The figure shows three views and two pictorial views of one solid part (mm, origin at its lowest corner). Answer the questions. A direction names the side the tool comes from. Round coordinates to 2 decimals unless told otherwise and drop trailing zeros. Write each loop counter-clockwise with the first axis right and the second up, starting at its lowest first coordinate (ties: lowest second). Pieces come first, ordered by that corner, then holes.
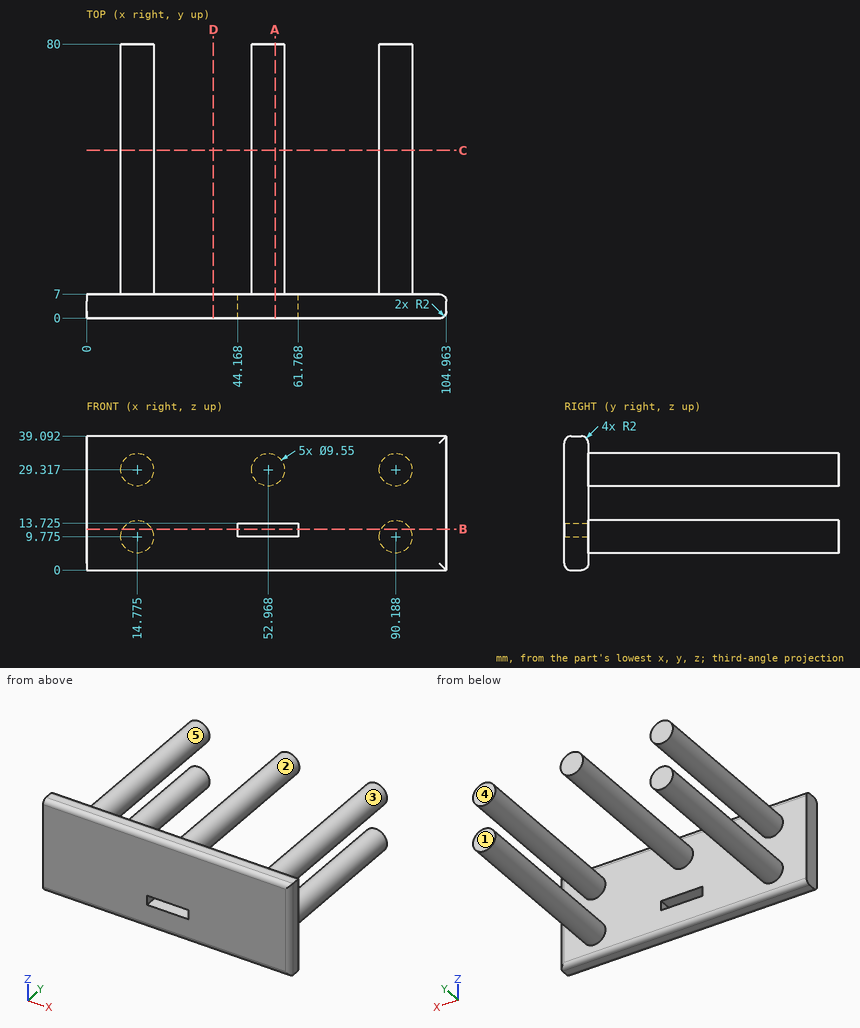
Q1. Determine the mould class of the marked faces 1, 2 and 3 for opening direction Z: pulls with the +Z half, pulls with the -Z half, needs draft (parallel to the pull), parting line crosses it, or undercut.
Verdict:
face 1: needs draft
face 2: parting line crosses it
face 3: undercut
Q2. Flat-ended cylindrical pins translate along their axes: pin 1 Ø12 at (y, z) = (28, 6) entering from +X; pin 2 Ø1 at (x, z) = (56.5, 22.5) entering from +Y; pin 3 Ø10 at (y, z) = (24, 6) entering from -X; pin 4 Ø4 at (y, z) = (38, 18.5) entering from +X. Find the tip coordinate at first contact, or state that the pin passes through.
Verdict:
pin 1: stops at x = 94.96
pin 2: stops at y = 7
pin 3: stops at x = 10
pin 4: passes through
Q3. Section B-B (z = 12) is taken. Determine the outline of the cut face in (x, y), then the cut area to 3 significant figures.
Verdict:
outline: (0, 0) - (44.17, 0) - (44.17, 7) - (19, 7) - (19, 80) - (10.55, 80) - (10.55, 7) - (0, 7) - close; (61.77, 0) - (102.96, 0) arc R2 ccw to (104.96, 2) - (104.96, 5) arc R2 ccw to (102.96, 7) - (94.41, 7) - (94.41, 80) - (85.96, 80) - (85.96, 7) - (61.77, 7) - close
area: 1,840 mm2
Q4. Section A-A (x = 55) is taken. Determine the outline of the cut face in (y, z) (1 decimal).
Verdict:
outline: (0, 2) arc R2 ccw to (2, 0) - (5, 0) arc R2 ccw to (7, 2) - (7, 9.8) - (0, 9.8) - close; (0, 13.7) - (7, 13.7) - (7, 25) - (80, 25) - (80, 33.6) - (7, 33.6) - (7, 37.1) arc R2 ccw to (5, 39.1) - (2, 39.1) arc R2 ccw to (0, 37.1) - close
Q5. Straight lines are drawn through the part: probe 1 along X at (y, z) = (72, 29); probe 2 along X at (y, z) = (64.5, 10) (1 decimal); probe 3 along X at (y, z) = (39, 32) (1 decimal). For each, find the intervals that lie inside material, in ascending order.
Verdict:
probe 1: x = 10.01 to 19.54, 48.2 to 57.73, 85.42 to 94.95
probe 2: x = 10 to 19.5, 85.4 to 95
probe 3: x = 10.8 to 18.7, 49 to 56.9, 86.2 to 94.1
Q6. Section C-C (y = 49) is taken. State how many separate pieces and enclosed holes the cut face has, then the cut area to 3 significant figures.
Verdict:
separate pieces: 5
enclosed holes: 0
area: 358 mm2
Q7. Which of the six approach directions +Z, -Z, +X, -X, +Y, -Y give full straight-line access (tool end or side, diameter ignored) to the marked faces 4 and 5?
Verdict:
face 4: +Z, -Z, +X, -X, +Y
face 5: +Y
Q8. Section D-D (x = 37) is taken. Determine the outline of the cut face in (y, z).
Verdict:
outline: (0, 2) arc R2 ccw to (2, 0) - (5, 0) arc R2 ccw to (7, 2) - (7, 37.09) arc R2 ccw to (5, 39.09) - (2, 39.09) arc R2 ccw to (0, 37.09) - close
